```python
from build123d import *

# Parameters (mm, degrees)
SKETCH1_W                = 15
SKETCH1_H                = 19
BOSS_EXTRUDE1_DEPTH      = 5
BOSS_EXTRUDE1_DEPTH_BACK = 5
CUT_EXTRUDE1_START       = -6
SKETCH2_R                = 2
CUT_EXTRUDE1_DEPTH       = 16
SKETCH5_R                = 2
CUT_EXTRUDE4_DEPTH       = 17
CUT_EXTRUDE4_DEPTH_BACK  = 17
SKETCH6_R                = 2
CUT_EXTRUDE5_DEPTH       = 17
CUT_EXTRUDE5_DEPTH_BACK  = 17
SKETCH10_W               = 9.46
SKETCH10_H               = 13.6
CUT_EXTRUDE6_DEPTH       = 6
CUT_EXTRUDE6_DEPTH_BACK  = 6
BOSS_EXTRUDE2_START      = -5
SKETCH7_R                = 5
SKETCH7_R_2              = 2.5
BOSS_EXTRUDE2_DEPTH      = 10
BOSS_EXTRUDE3_DEPTH      = 5
FILLET1_R                = 1.6
SKETCH11_W               = 12.27
SKETCH11_H               = 19
BOSS_EXTRUDE4_DEPTH      = 10
CHAMFER1_SIZE            = 1
SKETCH16_W               = 5.80562201
SKETCH16_H               = 3.2
CUT_EXTRUDE8_DEPTH       = 11.5
CUT_EXTRUDE9_DEPTH       = 11.5
TROU_TARAUD_M21_D        = 1.6
SKETCH24_W               = 11
SKETCH24_H               = 19
CUT_EXTRUDE10_DEPTH      = 2
CUT_EXTRUDE11_DEPTH      = 2
TROU_TARAUD_M2_51_D      = 2.05
TROU_TARAUD_M2_51_DEPTH  = 8.25
TROU_TARAUD_M2_51_TIP    = 0.615882135


with BuildPart() as part:
    # Sketch1 → Boss-Extrude1 (new body, two sides)
    with BuildSketch(Plane.XY) as boss_extrude1_sk:
        Rectangle(SKETCH1_W, SKETCH1_H)
    extrude(amount=BOSS_EXTRUDE1_DEPTH)
    extrude(boss_extrude1_sk.sketch, amount=-BOSS_EXTRUDE1_DEPTH_BACK)

    # Sketch2 → Cut-Extrude1 (cut)
    with BuildSketch(Plane.XY.offset(CUT_EXTRUDE1_START)):
        with Locations((-2.73, 6.8)):
            Circle(SKETCH2_R)
    cut_extrude1 = extrude(amount=CUT_EXTRUDE1_DEPTH, mode=Mode.SUBTRACT)

    # Mirror3: Cut-Extrude1 across plane
    add(cut_extrude1.mirror(Plane.ZX), mode=Mode.SUBTRACT)

    # Sketch5 → Cut-Extrude4 (cut, two sides)
    with BuildSketch(Plane.XY) as cut_extrude4_sk:
        with Locations((2.73, 6.8)):
            Circle(SKETCH5_R)
    extrude(amount=CUT_EXTRUDE4_DEPTH, mode=Mode.SUBTRACT)
    extrude(cut_extrude4_sk.sketch, amount=-CUT_EXTRUDE4_DEPTH_BACK, mode=Mode.SUBTRACT)

    # Sketch6 → Cut-Extrude5 (cut, two sides)
    with BuildSketch(Plane.XY) as cut_extrude5_sk:
        with Locations((2.73, -6.8)):
            Circle(SKETCH6_R)
    extrude(amount=CUT_EXTRUDE5_DEPTH, mode=Mode.SUBTRACT)
    extrude(cut_extrude5_sk.sketch, amount=-CUT_EXTRUDE5_DEPTH_BACK, mode=Mode.SUBTRACT)

    # Sketch10 → Cut-Extrude6 (cut, two sides)
    with BuildSketch(Plane.XY) as cut_extrude6_sk:
        Rectangle(SKETCH10_W, SKETCH10_H)
    extrude(amount=CUT_EXTRUDE6_DEPTH, mode=Mode.SUBTRACT)
    extrude(cut_extrude6_sk.sketch, amount=-CUT_EXTRUDE6_DEPTH_BACK, mode=Mode.SUBTRACT)



with BuildPart() as body_2:
    # Sketch7 → Boss-Extrude2 (new body)
    with BuildSketch(Plane.XY.offset(BOSS_EXTRUDE2_START)):
        Circle(SKETCH7_R)
        Circle(SKETCH7_R_2, mode=Mode.SUBTRACT)
    extrude(amount=BOSS_EXTRUDE2_DEPTH)


with BuildPart() as part_1:
    add(part.part)

    add(body_2.part)  # Boss-Extrude3 merges body 2
    # Sketch8 → Boss-Extrude3 (add, symmetric)
    with BuildSketch(Plane.XY):
        Polygon((0, 5), (-7.5, 5), (-7.5, 0), (-5, 0), align=None)
    boss_extrude3 = extrude(amount=BOSS_EXTRUDE3_DEPTH, both=True)

    # Mirror7: Boss-Extrude3 across plane
    add(boss_extrude3.mirror(Plane.ZX))

    # Fillet1
    fillet1_edges = [part_1.edges().sort_by_distance(p)[0] for p in [
        (-4.73, -5, 0),
        (-4.73, 5, 0),
    ]]
    fillet(fillet1_edges, radius=FILLET1_R)

    # Sketch11 → Boss-Extrude4 (add)
    with BuildSketch(Plane.XY.offset(5)):
        with Locations((10.865, 0)):
            Rectangle(SKETCH11_W, SKETCH11_H)
    extrude(amount=-BOSS_EXTRUDE4_DEPTH)

    # Chamfer1
    chamfer1_edges = [part_1.edges().sort_by_distance(p)[0] for p in [
        (17, 9.5, 0),
        (17, -9.5, 0),
        (-7.5, 9.5, 0),
        (-7.5, -9.5, 0),
    ]]
    chamfer(chamfer1_edges, length=CHAMFER1_SIZE)

    # Sketch16 → Cut-Extrude8 (cut)
    with BuildSketch(Plane.XY.offset(5)):
        with Locations((-0.227188995, 6.6)):
            Rectangle(SKETCH16_W, SKETCH16_H)
    cut_extrude8 = extrude(amount=-CUT_EXTRUDE8_DEPTH, mode=Mode.SUBTRACT)

    # Mirror8: Cut-Extrude8 across plane
    add(cut_extrude8.mirror(Plane.ZX), mode=Mode.SUBTRACT)

    # Sketch17 → Cut-Extrude9 (cut)
    with BuildSketch(Plane.XY.offset(5)):
        with BuildLine():
            ThreePointArc((2.678170763, -4.222250746), (5, 0), (2.678170763, 4.222250746))
            ThreePointArc((2.678170763, 4.222250746), (2.338473166, 5.740343478), (3.856565898, 6.080041075))
            ThreePointArc((3.856565898, 6.080041075), (7.2, 0), (3.856565898, -6.080041075))
            ThreePointArc((3.856565898, -6.080041075), (2.338473166, -5.740343478), (2.678170763, -4.222250746))
        make_face()
    extrude(amount=-CUT_EXTRUDE9_DEPTH, mode=Mode.SUBTRACT)

    # Trou taraudé M21 (through all)
    with Locations(Plane.XY.offset(5)):
        with Locations((14.5, 6.5), (14.5, -6.5), (9.5, 6.5), (9.5, -6.5), (9.5, 2.5), (14.5, 2.5), (14.5, -2.5), (9.5, -2.5)):
            Hole(TROU_TARAUD_M21_D / 2)

    # Sketch24 → Cut-Extrude10 (cut)
    with BuildSketch(Plane.XY.offset(5)):
        with Locations((11.5, 0)):
            Rectangle(SKETCH24_W, SKETCH24_H)
    extrude(amount=-CUT_EXTRUDE10_DEPTH, mode=Mode.SUBTRACT)

    # Sketch25 → Cut-Extrude11 (cut)
    with BuildSketch(Plane.XY.offset(5)):
        Polygon((17, -5.42836071), (4.73, -5.42836071), (6.865, 0), (4.73, 5.42836071), (17, 5.42836071), align=None)
    extrude(amount=-CUT_EXTRUDE11_DEPTH, mode=Mode.SUBTRACT)

    # Trou taraudé M2.51
    with Locations(Plane.ZY.offset(7.5)):
        with Locations((0, 0)):
            Hole(TROU_TARAUD_M2_51_D / 2, depth=TROU_TARAUD_M2_51_DEPTH)
            with Locations((0, 0, -(TROU_TARAUD_M2_51_DEPTH + TROU_TARAUD_M2_51_TIP / 2))):  # 118° drill point
                Cone(0, TROU_TARAUD_M2_51_D / 2, TROU_TARAUD_M2_51_TIP, mode=Mode.SUBTRACT)


solid = part_1.part
```
Read the model definition and answer for the solid it produces. Units are mm, in the model's axes. A direction names the side the tool comes from. Give positions to 0.01 mm unless a question says otherwise; leave off trailing zeros. Loops run counter-clockwise (first coordinate to the right, second up) from the corner with the lowest first, then second, coordinate; pieces in that order, holes last.
Item 1: Find the intervals of material crossed by line 1 along Y through (x, z) = (14.5, 1); line 2 along Y through (x, z) = (0, -3.5); line 3 along Y through (x, z) = (4, 3), in increasing order.
Item 2: The part is cut by section B-B (y = -3). Write down the section's boundary in (x, z), and give its area (3 significant figures).
Item 3: The part is cut by section C-C (x = 9.5). Write down the section's boundary in (y, z).
Item 4: Each of these flat-tipped pins is pushed along its axis until it touches: pin 1 Ø0.6 at (y, z) = (-8, 4.5) entering from +X; pin 2 Ø1.8 at (x, y) = (14.5, 2.5) entering from -Z; pin 3 Ø1 at (x, y) = (9.5, -6.5) entering from +Z; pin 4 Ø1.6 at (y, z) = (0, 0) entering from -X. Where does it stop, or does it pass through?
Item 5: The mould has two halves that part along X. Classify faces 1 (the flat face through (5, -5.428, 4)), 2 (the flat face through (-7, -9, 0)), 3 (the cylindrical face through (10.09, -1.96, -1.06)): released by +X, released by -X, zero draft, split by the parting line, or undercut.
Item 6: For faces 4 (the cylindrical face through (-4.25, 5.46, 0.07)), 5 (the flat face through (6, -7, 4)), 6 (the flat face through (5, -9.5, 0)), determine the directions among +Z, -Z, +X, -X, +Y, -Y from which every point of the face is accessible in a straight line to the end or side of a thin tool.
Item 7: The part is cut by section D-D (y = 4). Write down the section's boundary in (x, z).
Item 8: The part is cut by section A-A (z = 3.5). Write down the section's boundary in (x, y), and give its area (3 significant figures).
Taken from the geometry:
1. line 1: y = -9.5 to -7.3, -5.7 to -3.3, -1.7 to 1.7, 3.3 to 5.7, 7.3 to 9.5
1. line 2: y = -9.5 to -8.2, -5 to -2.5, 2.5 to 5, 8.2 to 9.5
1. line 3: y = -9.5 to -8.35, -3 to 3, 8.35 to 9.5
2. outline: (-7.5, -5) - (4, -5) - (4, 5) - (-7.5, 5) - close; (6.55, -5) - (8.88, -5) - (8.88, 3) - (6.55, 3) - close; (10.12, -5) - (13.88, -5) - (13.88, 3) - (10.12, 3) - close; (15.12, -5) - (17, -5) - (17, 3) - (15.12, 3) - close
2. area: 179 mm2
3. outline: (-9.5, -5) - (-7.3, -5) - (-7.3, 3) - (-9.5, 3) - close; (-5.7, -5) - (-3.3, -5) - (-3.3, 3) - (-5.7, 3) - close; (-1.7, -5) - (1.7, -5) - (1.7, 3) - (-1.7, 3) - close; (3.3, -5) - (5.7, -5) - (5.7, 3) - (3.3, 3) - close; (7.3, -5) - (9.5, -5) - (9.5, 3) - (7.3, 3) - close
4. pin 1: stops at x = 6
4. pin 2: stops at z = -5
4. pin 3: passes through
4. pin 4: stops at x = 2.37
5. face 1: zero draft
5. face 2: released by -X
5. face 3: undercut
6. face 4: +Z, -Z
6. face 5: +Z, +X, +Y, -Y
6. face 6: +Z, -Z, +X, -X, -Y
7. outline: (-7.5, -5) - (3, -5) - (3, 5) - (-7.5, 5) - close; (5.99, -5) - (17, -5) - (17, 3) - (5.99, 3) - close
8. outline: (-7.5, -8.5) - (-6.5, -9.5) - (6, -9.5) - (6, -5.43) - (4.73, -5.43) - (4.73, -6.8) arc R2 cw to (1.3, -8.2) - (-1.3, -8.2) arc R2 cw to (-4.73, -6.8) - (-4.73, -6.6) arc R1.6 cw to (-3.13, -5) - (0, -5) arc R5 ccw to (0, 5) - (-3.13, 5) arc R1.6 cw to (-4.73, 6.6) - (-4.73, 6.8) arc R2 cw to (-1.3, 8.2) - (1.3, 8.2) arc R2 cw to (4.73, 6.8) - (4.73, 5.43) - (6, 5.43) - (6, 9.5) - (-6.5, 9.5) - (-7.5, 8.5) - close; hole circle Ø5 at (0, 0)
8. area: 151 mm2
